Autodesk Inventor part; units mm, degrees
ref_plane "Work Plane1" through (0, 0, 0) normal (0, 0, 1) x (1, 0, 0)
ref_plane "YZ Plane" through (0, 0, 0) normal (1, 0, 0) x (0, 1, 0)
ref_plane "XZ Plane" through (0, 0, 0) normal (0, 1, 0) x (-1, 0, 0)
ref_plane "Work Plane1" through (0, 0, 0) normal (0, 0, 1) x (1, 0, 0)
sketch "Sketch1" plane through (0, 0, 0) normal (0, 0, 1) x (1, 0, 0)
  line L0 (-533.4, -800.8554) -> (-63.844, -965.2)
  line L1 (-533.4, -965.2) -> (-25.4, -965.2)
  line L2 (-25.4, -951.7446) -> (-494.956, -787.4)
  line L3 (-533.4, -990.6) -> (-25.4, -990.6)
  line L4 (-25.4, -787.4) -> (-25.4, -1498.6)
  line L5 (0, -787.4) -> (0, -1498.6)
  arc A0 (-40.1687, -977.9762) -> (-36.0313, -977.9762) centre (-38.1, -977.9) ccw
  arc A1 (-36.0313, -977.8238) -> (-40.1687, -977.8238) centre (-38.1, -977.9) ccw
  arc A2 (-65.5687, -977.9762) -> (-61.4313, -977.9762) centre (-63.5, -977.9) ccw
  arc A3 (-61.4313, -977.8238) -> (-65.5687, -977.8238) centre (-63.5, -977.9) ccw
  line L6 (-116.3687, -977.8238) -> (-137.6313, -977.8238)
  arc A4 (-12.7762, -975.8313) -> (-12.7762, -979.9687) centre (-12.7, -977.9) ccw
  arc A5 (-12.6238, -979.9687) -> (-12.6238, -975.8313) centre (-12.7, -977.9) ccw
  arc A6 (-12.7762, -950.4313) -> (-12.7762, -954.5687) centre (-12.7, -952.5) ccw
  arc A7 (-12.6238, -954.5687) -> (-12.6238, -950.4313) centre (-12.7, -952.5) ccw
  arc A8 (-12.7762, -925.0313) -> (-12.7762, -929.1687) centre (-12.7, -927.1) ccw
  arc A9 (-12.6238, -929.1687) -> (-12.6238, -925.0313) centre (-12.7, -927.1) ccw
  circle A10 centre (-31.3935, -963.1023) radius 2.032
  circle A11 centre (-55.3675, -954.7114) radius 2.032
  circle A12 centre (-79.3415, -946.3205) radius 2.032
  arc A13 (-12.7762, -899.6313) -> (-12.7762, -903.7687) centre (-12.7, -901.7) ccw
  arc A14 (-12.6238, -903.7687) -> (-12.6238, -899.6313) centre (-12.7, -901.7) ccw
  arc A15 (-90.9687, -977.9762) -> (-86.8313, -977.9762) centre (-88.9, -977.9) ccw
  arc A16 (-86.8313, -977.8238) -> (-90.9687, -977.8238) centre (-88.9, -977.9) ccw
  line L7 (-12.7, -901.7) -> (-12.7, -876.3) construction
  line L8 (-25.4, -889) -> (0, -889) construction
  line L9 (0, -889) -> (-25.4, -889)
  line L10 (-88.9, -977.9) -> (-114.3, -977.9) construction
  line L11 (-101.6, -990.6) -> (-101.6, -965.2)
  line L12 (-101.6, -990.6) -> (0, -990.6)
  line L13 (0, -990.6) -> (0, -889)
  line L14 (-25.4, -889) -> (-25.4, -951.7446)
  line L15 (-101.6, -965.2) -> (-63.844, -965.2)
  line L16 (-79.3415, -946.3205) -> (-103.3155, -937.9296) construction
  line L17 (-95.524, -954.112) -> (-87.1331, -930.138) construction
  line L18 (-87.1331, -930.138) -> (-95.524, -954.112)
  line L19 (-95.524, -954.112) -> (-63.844, -965.2)
  line L20 (-87.1331, -930.138) -> (-25.4, -951.7446)
  circle A17 centre (-12.7, -901.7) radius 2.0701
  circle A18 centre (-12.7, -927.1) radius 2.0701
  circle A19 centre (-12.7, -952.5) radius 2.0701
  circle A20 centre (-12.7, -977.9) radius 2.0701
  circle A21 centre (-38.1, -977.9) radius 2.0701
  circle A22 centre (-63.5, -977.9) radius 2.0701
  circle A23 centre (-88.9, -977.9) radius 2.0701
  circle A24 centre (-79.3415, -946.3205) radius 2.032
  circle A25 centre (-55.3675, -954.7114) radius 2.032
  circle A26 centre (-31.3935, -963.1023) radius 2.032
  point P0 (0, 0)
  point P1 (-12.7762, -903.7687)
  point P2 (-12.6238, -899.6313)
  point P3 (-12.7762, -929.1687)
  point P4 (-12.6238, -925.0313)
  point P5 (-12.7762, -954.5687)
  point P6 (-12.6238, -950.4313)
  point P7 (-12.7762, -979.9687)
  point P8 (-12.6238, -975.8313)
  point P9 (-86.8313, -977.9762)
  point P10 (-40.1687, -977.8238)
  point P11 (-36.0313, -977.9762)
  point P12 (-25.4, -990.6)
  dimension "d0" = 25.4
  dimension "d1" = 25.4
  dimension "d2" = 25.4
extrude "Extrusion1" add sketch "Sketch1" along normal blind 3.175
properties part number "arrow bracket (70.1 and 19.29 degrees)"
Can you work these out from the model? Positions are in its coordinate system, mm. A direction names the side the tool comes from. Round coordinates to 2 decimals unless told otherwise and drop trailing zeros. Loops run counter-clockwise (first coordinate to the right, second up) from the corner with the lowest first, then second, coordinate; pieces in that order, holes last. Notation, with made-up numbers: (78.5, 86) - (85.5, 86) arc R4 ccw to (85.5, 93) - close; hole circle Ø9 at (50.25, 10.5). An arc over 180 degrees is marked (long way). Answer in a Markdown table with one row per item. Add a question column.
Q1. Which directions (+Z, -Z, +X, -X, +Y, -Y) give clear straight access to the entire face, cutting with the end or side of a thin tool? Please do faces 4 (the flat face through (-55.834, -941.093, 1.565)), 5 (the flat face through (-83, -965.2, 2)), 6 (the flat face through (-91.27, -941.96, 1.57)).
Q2. I want a section at D-D on z = 0.85. Count the separate pieces of the cut face and the enclosed holes in it, and give its area (3 significant figures).
Q3. I want a section at C-C on x = -38.1. List the corners of the cut face in (y, z) for me (3 decimals).
Q4. I need wall thicknesses on L1, parallel to Y at x = -64.5, z = 1.3; L2, parallel to X at y = -915, z = 2.15; L3, parallel to Y at x = -31, z = 1.2. Which ranges of each line are inside material? Lowest first, please.
Q5. For pin 1 Ø1 at (y, z) = (-924.5, 3) entering from -X; pin 2 Ø3.5 at (x, y) = (-79.34, -946.32) entering from -Z, each with a flat end and sliding along its axis, tell me the tip position at first contact or that it passes through.
Q6. I want a section at A-A on y = -927.1. List the corners of the cut face in (x, z) for me (3 decimals), and give its area (3 significant figures).
Q7. We'd pull the mould along X, two halves only. Please class faces 1 (the flat face through (-52, -990.6, 2)), 2 (the flat face through (-25.4, -920, 2)), 3 (the flat face through (0, -939, 2)): pulls with the +X half, pulls with the -X half, needs draft (parallel to the pull), parting line crosses it, or undercut.
Q8. I want a section at B-B on x = -88.9. List the corners of the cut face in (y, z) for me (3 decimals).
A:
| question | item | result |
|---|---|---|
| 1 | face 4 | +Z, -Z, +Y |
| 1 | face 5 | +Z, -Z, -X |
| 1 | face 6 | +Z, -Z, -X, +Y |
| 2 | separate pieces | 1 |
| 2 | enclosed holes | 10 |
| 2 | area | 5,900 mm^2 |
| 3 | outline | (-990.6, 0) - (-979.97, 0) - (-979.97, 3.175) - (-990.6, 3.175) - close; (-975.83, 0) - (-947.3, 0) - (-947.3, 3.175) - (-975.83, 3.175) - close |
| 4 | L1 | -990.6 to -979.71, -976.09 to -965.2, -964.97 to -938.06 |
| 4 | L2 | -25.4 to 0 |
| 4 | L3 | -990.6 to -965.1, -961.11 to -949.78 |
| 5 | pin 1 | x = -25.4 |
| 5 | pin 2 | through |
| 6 | outline | (-25.4, 0) - (-14.77, 0) - (-14.77, 3.175) - (-25.4, 3.175) - close; (-10.63, 0) - (0, 0) - (0, 3.175) - (-10.63, 3.175) - close |
| 6 | area | 67.5 mm^2 |
| 7 | face 1 | needs draft |
| 7 | face 2 | undercut |
| 7 | face 3 | pulls with the +X half |
| 8 | outline | (-990.6, 0) - (-979.97, 0) - (-979.97, 3.175) - (-990.6, 3.175) - close; (-975.83, 0) - (-965.2, 0) - (-965.2, 3.175) - (-975.83, 3.175) - close; (-956.43, 0) - (-935.186, 0) - (-935.186, 3.175) - (-956.43, 3.175) - close |
